Build history of the part. All positions in model axes, mm. A direction names the side the tool comes from. Round coordinates to 2 decimals unless told otherwise and drop trailing zeros. Write each loop counter-clockwise with the first axis right and the second up, starting at its lowest first coordinate (ties: lowest second). Pieces come first, ordered by that corner, then holes. Notation, with made-up numbers: (4, 49.5) -> (62, 49.5) arc R13 cw to (62, 66.5) -> close; hole circle Ø1 at (12.5, 8.25). An arc over 180 degrees is marked (long way). Answer as CSV lines item,"result".
from build123d import *

# Parameters (mm, degrees)
SKETCH2_R               = 1.5
BOSS_EXTRUDE2_DEPTH     = 6
SKETCH3_W               = 22
SKETCH3_H               = 38
BOSS_EXTRUDE3_DEPTH     = 12
CUT_EXTRUDE1_DEPTH      = 50.969990995
CUT_EXTRUDE1_DEPTH_BACK = 50.969990995
SKETCH5_R               = 1.55


with BuildPart() as part:
    # Sketch2 → Boss-Extrude2 (new body)
    with BuildSketch(Plane.XY):
        with BuildLine():
            Line((8.544155877, 19), (-8.544155877, 19))
            ThreePointArc((-8.544155877, 19), (-14.284407363, 20.141807012), (-19.150757595, 23.393398282))
            Line((-19.150757595, 23.393398282), (-21.878679656, 26.121320344))
            ThreePointArc((-21.878679656, 26.121320344), (-26.121320344, 26.121320344), (-26.121320344, 21.878679656))
            Line((-26.121320344, 21.878679656), (-23.393398282, 19.150757595))
            ThreePointArc((-23.393398282, 19.150757595), (-20.141807012, 14.284407363), (-19, 8.544155877))
            Line((-19, 8.544155877), (-19, -8.544155877))
            ThreePointArc((-19, -8.544155877), (-20.141807012, -14.284407363), (-23.393398282, -19.150757595))
            Line((-23.393398282, -19.150757595), (-26.121320344, -21.878679656))
            ThreePointArc((-26.121320344, -21.878679656), (-26.121320344, -26.121320344), (-21.878679656, -26.121320344))
            Line((-21.878679656, -26.121320344), (-19.150757595, -23.393398282))
            ThreePointArc((-19.150757595, -23.393398282), (-14.284407363, -20.141807012), (-8.544155877, -19))
            Line((-8.544155877, -19), (8.544155877, -19))
            ThreePointArc((8.544155877, -19), (14.284407363, -20.141807012), (19.150757595, -23.393398282))
            Line((19.150757595, -23.393398282), (21.878679656, -26.121320344))
            ThreePointArc((21.878679656, -26.121320344), (26.121320344, -26.121320344), (26.121320344, -21.878679656))
            Line((26.121320344, -21.878679656), (23.393398282, -19.150757595))
            ThreePointArc((23.393398282, -19.150757595), (20.141807012, -14.284407363), (19, -8.544155877))
            Line((19, -8.544155877), (19, 8.544155877))
            ThreePointArc((19, 8.544155877), (20.141807012, 14.284407363), (23.393398282, 19.150757595))
            Line((23.393398282, 19.150757595), (26.121320344, 21.878679656))
            ThreePointArc((26.121320344, 21.878679656), (26.121320344, 26.121320344), (21.878679656, 26.121320344))
            Line((21.878679656, 26.121320344), (19.150757595, 23.393398282))
            ThreePointArc((19.150757595, 23.393398282), (14.284407363, 20.141807012), (8.544155877, 19))
        make_face()
        with Locations((15, 15)):
            Circle(SKETCH2_R, mode=Mode.SUBTRACT)
        with Locations((24, 24)):
            Circle(SKETCH2_R, mode=Mode.SUBTRACT)
        with Locations((24, -24)):
            Circle(SKETCH2_R, mode=Mode.SUBTRACT)
        with Locations((15, -15)):
            Circle(SKETCH2_R, mode=Mode.SUBTRACT)
        with Locations((-24, -24)):
            Circle(SKETCH2_R, mode=Mode.SUBTRACT)
        with Locations((-15, -15)):
            Circle(SKETCH2_R, mode=Mode.SUBTRACT)
        with Locations((-24, 24)):
            Circle(SKETCH2_R, mode=Mode.SUBTRACT)
        with Locations((-15, 15)):
            Circle(SKETCH2_R, mode=Mode.SUBTRACT)
    extrude(amount=BOSS_EXTRUDE2_DEPTH)

    # Sketch3 → Boss-Extrude3 (add)
    with BuildSketch(Plane.XY.offset(6)):
        Rectangle(SKETCH3_W, SKETCH3_H)
    extrude(amount=BOSS_EXTRUDE3_DEPTH)

    # Sketch5 → Cut-Extrude1 (cut, two sides: drawn at the far end of the back side and taken through both)
    with BuildSketch(Plane.ZY.offset(11).offset(-CUT_EXTRUDE1_DEPTH_BACK)):
        with Locations(Location((13, -10, 0), (0, 0, 270))):
            Circle(SKETCH5_R)
        with Locations(Location((13, 10, 0), (0, 0, 270))):
            Circle(SKETCH5_R)
    extrude(amount=CUT_EXTRUDE1_DEPTH + CUT_EXTRUDE1_DEPTH_BACK, mode=Mode.SUBTRACT)


solid = part.part
1. Mould opens along Y. For faces 5 (the flat face through (-11, 0, 12)), 6 (the cylindrical face through (14.361, 20.174, 2.958)), 7 (the flat face through (-24.74, -20.5, 2.96)) say: +Y half, -Y half, draft (parallel to the pull), parting line (faces both ways), or undercut.
Results found:
face 5,"draft"
face 6,"+Y half"
face 7,"undercut"
2. Drop flat-ended pins along their axis: pin 1 Ø2.5 at (x, y) = (15, 15) entering from -Z; pin 2 Ø5 at (y, z) = (0, 4.5) entering from +X; pin 3 Ø5 at (y, z) = (10, 13) entering from -X; pin 4 Ø5.5 at (x, z) = (-1, 7.5) entering from -Y. Give the stop position or say it passes through.
Results found:
pin 1,"passes through"
pin 2,"stops at x = 19"
pin 3,"stops at x = -11"
pin 4,"stops at y = -19"
3. Cut at B-B, the plane x = 15. Write the cut outline in (y, z).
Results found:
outline,"(-20.46, 0) -> (-16.5, 0) -> (-16.5, 6) -> (-20.46, 6) -> close; (-13.5, 0) -> (13.5, 0) -> (13.5, 6) -> (-13.5, 6) -> close; (16.5, 0) -> (20.46, 0) -> (20.46, 6) -> (16.5, 6) -> close"
4. Cut at D-D, the plane x = 1.5. Write the cut outline in (y, z).
Results found:
outline,"(-19, 0) -> (19, 0) -> (19, 18) -> (-19, 18) -> close; hole circle Ø3.1 at (-10, 13); hole circle Ø3.1 at (10, 13)"
5. Probe line 1 along Y through (x, z) = (15, 4.2); line 2 along Z through (x, y) = (1, 10); line 3 along X through (y, z) = (-8.5, 7.75). List the from-to ranges inside material, lowest first.
Results found:
line 1,"y = -20.46 to -16.5, -13.5 to 13.5, 16.5 to 20.46"
line 2,"z = 0 to 11.45, 14.55 to 18"
line 3,"x = -11 to 11"
6. Which spindle directions (+Z, -Z, +X, -X, +Y, -Y) get a long thin tool onto all of the face, cutting with end or side? Do faces 1 (the flat face through (24.74, 20.5, 2.96)), 2 (the flat face through (0, -19, 9)), 3 (the flat face through (0, 19, 9)), 4 (the flat face through (-20.5, 24.74, 2.96)). Say none if no direction does.
Results found:
face 1,"+Z, -Z, +X"
face 2,"+Z, -Y"
face 3,"+Z, +Y"
face 4,"+Z, -Z, +Y"
7. Cut at A-A, the plane z = 2.5. Count the separate pieces of the cut face and the enclosed holes in it, then the cut area to 3 significant figures.
Results found:
separate pieces,"1"
enclosed holes,"8"
area,"1,690 mm2"
8. Cut at C-C, the plane y = 10. Write the cut outline in (x, z), then the cut area to 3 significant figures.
Results found:
outline,"(-19.07, 0) -> (19.07, 0) -> (19.07, 6) -> (11, 6) -> (11, 11.45) -> (-11, 11.45) -> (-11, 6) -> (-19.07, 6) -> close; (-11, 14.55) -> (11, 14.55) -> (11, 18) -> (-11, 18) -> close"
area,"425 mm2"
